Here's how the part is built. I have some questions about the finished solid (model axes, mm). Face numbers are marked on the shaded views. Coordinates: 2 decimals unless noted, no trailing zeros. Write each loop counter-clockwise with the first axis right and the second up, starting at its lowest first coordinate (ties: lowest second). Pieces come first, ordered by that corner, then holes. Notation, with made-up numbers: (-10, -31) -> (13, -31) arc R37 ccw to (13, 5) -> close; hole circle Ø1 at (69, 49). An arc over 180 degrees is marked (long way). Put each result on its own line as item: value.
```python
from build123d import *

# Parameters (mm, degrees)
SKETCH_1_R             = 13.5
EXTRUDE_1_DEPTH        = 28.8
SKETCH_2_R             = 12.16
EXTRUDE_2_DEPTH        = 18
SKETCH_3_R             = 4
CUT_EXTRUDE_1_DEPTH    = 0.5
SKETCH_4_R             = 3.24
EXTRUDE_3_DEPTH        = 2.06
FILLET_1_R             = 0.1
FILLET_2_R             = 1
EXTRUDE_4_DEPTH        = 0.5
SKETCH_6_W             = 2.145218315
SKETCH_6_H             = 0.731898013
SKETCH_6_W_2           = 2.145218314
SKETCH_6_H_2           = 0.731898014
EXTRUDE_5_DEPTH        = 3.5
FILLET_3_R             = 1
CUT_EXTRUDE_2_DEPTH    = 2.7
PATTERN_LINEAR_1_COUNT = 2
PATTERN_LINEAR_1_PITCH = 9
SKETCH_10_R            = 0.323097308
CUT_EXTRUDE_3_DEPTH    = 2.7
SKETCH_13_R            = 0.255477279
CUT_EXTRUDE_4_DEPTH    = 2.7
CUT_EXTRUDE_5_DEPTH    = 2


with BuildPart() as part:
    # 草图1 → 凸台-拉伸1 (new body)
    with BuildSketch(Plane.XY):
        Circle(SKETCH_1_R)
    extrude(amount=EXTRUDE_1_DEPTH)

    # 草图2 → 凸台-拉伸2 (add)
    with BuildSketch(Plane.XY.offset(28.8)):
        Circle(SKETCH_2_R)
    extrude(amount=EXTRUDE_2_DEPTH)

    # 草图3 → 切除-拉伸1 (cut)
    with BuildSketch(Plane.XY.offset(46.8)):
        Circle(SKETCH_3_R)
    extrude(amount=-CUT_EXTRUDE_1_DEPTH, mode=Mode.SUBTRACT)

    # 草图4 → 凸台-拉伸3 (add)
    with BuildSketch(Plane.XY.offset(46.3)):
        Circle(SKETCH_4_R)
    extrude(amount=EXTRUDE_3_DEPTH)

    # 圆角1
    fillet_1_edges = [part.edges().sort_by_distance(p)[0] for p in [
        (-4, 0, 46.8),
    ]]
    fillet(fillet_1_edges, radius=FILLET_1_R)

    # 圆角2
    fillet_2_edges = [part.edges().sort_by_distance(p)[0] for p in [
        (-3.24, 0, 48.36),
    ]]
    fillet(fillet_2_edges, radius=FILLET_2_R)

    # 草图5 → 凸台-拉伸4 (add)
    with BuildSketch(Plane.XY.offset(46.8)):
        with BuildLine():
            Line((-7.16, 2), (-7.16, -2))
            ThreePointArc((-7.16, -2), (-8.83, -3.67), (-10.5, -2))
            Line((-10.5, -2), (-10.5, 2))
            ThreePointArc((-10.5, 2), (-8.83, 3.67), (-7.16, 2))
        make_face()
        with BuildLine():
            Line((7.16, 2), (7.16, -2))
            ThreePointArc((7.16, -2), (8.83, -3.67), (10.5, -2))
            Line((10.5, -2), (10.5, 2))
            ThreePointArc((10.5, 2), (8.83, 3.67), (7.16, 2))
        make_face()
    extrude(amount=EXTRUDE_4_DEPTH)

    # 草图6 → 凸台-拉伸5 (add)
    with BuildSketch(Plane.XY.offset(47.3)):
        with Locations((-8.86959666, -1.801422961)):
            Rectangle(SKETCH_6_W, SKETCH_6_H)
        with Locations((8.784288178, 1.946399625)):
            Rectangle(SKETCH_6_W_2, SKETCH_6_H_2)
    extrude(amount=EXTRUDE_5_DEPTH)

    # 圆角3
    fillet_3_edges = [part.edges().sort_by_distance(p)[0] for p in [
        (7.711679021, 1.946399625, 50.8),
        (9.856897335, 1.946399625, 50.8),
        (-9.942205817, -1.80142296, 50.8),
        (-7.796987502, -1.80142296, 50.8),
    ]]
    fillet(fillet_3_edges, radius=FILLET_3_R)

    # 草图7 → 切除-拉伸2 (cut)
    with BuildSketch(Plane(origin=(0, 0, 0), x_dir=(-1, 0, 0), z_dir=(0, 0, -1))):
        with BuildLine():
            Line((1.85, 16), (1.85, 11))
            ThreePointArc((1.85, 11), (0, 9.15), (-1.85, 11))
            Line((-1.85, 11), (-1.85, 16))
            ThreePointArc((-1.85, 16), (0, 17.85), (1.85, 16))
        make_face()
        with BuildLine():
            Line((12.931406461, -9.602146997), (8.601279442, -7.102146997))
            ThreePointArc((8.601279442, -7.102146997), (7.924132445, -4.575), (10.451279442, -3.897853003))
            Line((10.451279442, -3.897853003), (14.781406461, -6.397853003))
            ThreePointArc((14.781406461, -6.397853003), (15.458553458, -8.925), (12.931406461, -9.602146997))
        make_face()
        with BuildLine():
            Line((-14.781406461, -6.397853003), (-10.451279442, -3.897853003))
            ThreePointArc((-10.451279442, -3.897853003), (-7.924132445, -4.575), (-8.601279442, -7.102146997))
            Line((-8.601279442, -7.102146997), (-12.931406461, -9.602146997))
            ThreePointArc((-12.931406461, -9.602146997), (-15.458553458, -8.925), (-14.781406461, -6.397853003))
        make_face()
    extrude(amount=-CUT_EXTRUDE_2_DEPTH, mode=Mode.SUBTRACT)

    # 草图9 → 旋转1 (revolve)
    with BuildSketch(Plane(origin=(0, 0, 0), x_dir=(1, 0, 0), z_dir=(0, 1, 0))):
        Polygon((0, 7), (0, 0), (-2.905653035, 0), (-2, 0.905653035), (-2, 3.949637413), (-0.890685833, 5.05895158), (-2, 5.05895158), (-2, 5.636365699), (-0.636365699, 7), align=None)
    revolve_1 = revolve(axis=Axis((0, 0, -8.873463159), (0, 0, 1)))

    # 阵列(线性)1: 旋转1 ×2
    with Locations(*[(0, -i * PATTERN_LINEAR_1_PITCH, 0) for i in range(1, PATTERN_LINEAR_1_COUNT)]):
        add(revolve_1)

    # 草图10 → 切除-拉伸3 (cut)
    with BuildSketch(Plane(origin=(0, 0, -7), x_dir=(-1, 0, 0), z_dir=(0, 0, -1))):
        Circle(SKETCH_10_R)
    extrude(amount=-CUT_EXTRUDE_3_DEPTH, mode=Mode.SUBTRACT)

    # 草图13 → 切除-拉伸4 (cut)
    with BuildSketch(Plane(origin=(0, 0, -7), x_dir=(-1, 0, 0), z_dir=(0, 0, -1))):
        with Locations((0, -9)):
            Circle(SKETCH_13_R)
    extrude(amount=-CUT_EXTRUDE_4_DEPTH, mode=Mode.SUBTRACT)

    # 草图14 → 切除-拉伸5 (cut)
    with BuildSketch(Plane(origin=(0, 0, 0), x_dir=(-1, 0, 0), z_dir=(0, 0, -1))):
        with BuildLine():
            Line((-0.52608989, 4.972245914), (-0.52608989, 3.431742925))
            ThreePointArc((-0.52608989, 3.431742925), (0, 2.905653035), (0.52608989, 3.431742925))
            Line((0.52608989, 3.431742925), (0.52608989, 4.972245914))
            ThreePointArc((0.52608989, 4.972245914), (2.219187285, 4.480536552), (3.636363636, 3.431742925))
            ThreePointArc((3.636363636, 3.431742925), (4.343174293, 3.411280854), (4.363636364, 4.11809151))
            ThreePointArc((4.363636364, 4.11809151), (0, 6), (-4.363636364, 4.11809151))
            ThreePointArc((-4.363636364, 4.11809151), (-4.343174293, 3.411280854), (-3.636363636, 3.431742925))
            ThreePointArc((-3.636363636, 3.431742925), (-2.219187285, 4.480536552), (-0.52608989, 4.972245914))
        make_face()
        with BuildLine():
            Line((2.708931608, -2.171478672), (4.04304633, -2.941730166))
            ThreePointArc((4.04304633, -2.941730166), (2.770664835, -4.16214084), (1.153794734, -4.865054749))
            ThreePointArc((1.153794734, -4.865054749), (0.782668733, -5.466939697), (1.384553681, -5.838065699))
            ThreePointArc((1.384553681, -5.838065699), (5.196152423, -3), (5.748190045, 1.719974189))
            ThreePointArc((5.748190045, 1.719974189), (5.125843025, 2.055658843), (4.790158371, 1.433311824))
            ThreePointArc((4.790158371, 1.433311824), (4.989852119, -0.318395712), (4.56913622, -2.030515748))
            Line((4.56913622, -2.030515748), (3.235021497, -1.260264253))
            ThreePointArc((3.235021497, -1.260264253), (2.516369343, -1.452826518), (2.708931608, -2.171478672))
        make_face()
        with BuildLine():
            Line((-3.235021497, -1.260264253), (-4.56913622, -2.030515748))
            ThreePointArc((-4.56913622, -2.030515748), (-4.989852119, -0.318395712), (-4.790158371, 1.433311824))
            ThreePointArc((-4.790158371, 1.433311824), (-5.125843025, 2.055658843), (-5.748190045, 1.719974189))
            ThreePointArc((-5.748190045, 1.719974189), (-5.196152423, -3), (-1.384553681, -5.838065699))
            ThreePointArc((-1.384553681, -5.838065699), (-0.782668733, -5.466939697), (-1.153794734, -4.865054749))
            ThreePointArc((-1.153794734, -4.865054749), (-2.770664835, -4.16214084), (-4.04304633, -2.941730166))
            Line((-4.04304633, -2.941730166), (-2.708931608, -2.171478672))
            ThreePointArc((-2.708931608, -2.171478672), (-2.516369343, -1.452826518), (-3.235021497, -1.260264253))
        make_face()
    extrude(amount=-CUT_EXTRUDE_5_DEPTH, mode=Mode.SUBTRACT)


solid = part.part
```
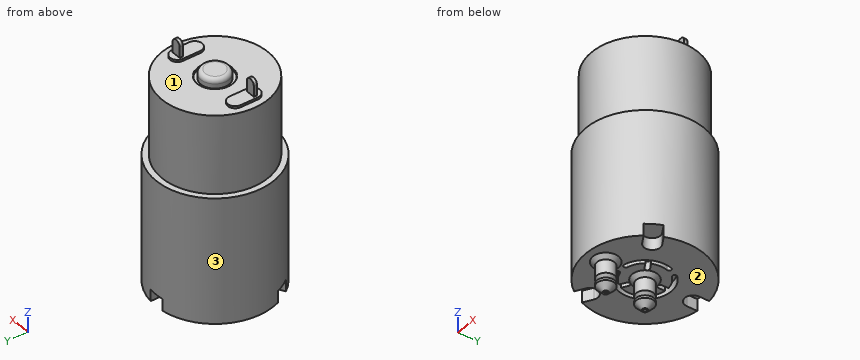
Item 1: If we mould it in two halves opening along X, with no side actions, what happens to the marked faces 1, 2 and 3? For each: released by +X, released by -X, zero draft, split by the parting line, or undercut.
Output:
face 1: undercut
face 2: zero draft
face 3: split by the parting line
Item 2: Imagine slicing it at A-A on z = 24.5. Write out the boundary of the cut face in (x, y).
Output:
outline: circle Ø27 at (0, 0)
Item 3: Please list where these lines run through material, in increasing order: line 1 along Y through (x, z) = (0, -5.4); line 2 along X through (y, z) = (0, 1); line 3 along Y through (x, z) = (0, 46.55). Write a range as from..to.
Output:
line 1: y = -11..-9.26, -8.74..-7, -2..-0.32, 0.32..2
line 2: x = -13.5..-6, -5..5, 6..13.5
line 3: y = -12.16..-4, -3.24..3.24, 4..12.16
Item 4: For P1, Ø1.5, axis at x = 0, y = -10, coming from the +Z side; P2, Ø4, axis at x = -5, y = 1.5, coming from the -Z side; P3, Ø12, axis at x = -7, y = 7.5, coming from the +Z side, each with a flat end and sliding along its axis, tell me the tip position at first contact or that it passes through.
Output:
P1: stops at z = 46.8
P2: stops at z = 0
P3: stops at z = 47.3
